from build123d import *

# Parameters (mm, degrees)
SKETCH1_W           = 2.54
SKETCH1_H           = 8.5
BOSS_EXTRUDE1_DEPTH = 1.52
SKETCH_1_W          = 0.8
SKETCH_1_H          = 1.54
CUT_EXTRUDE_1_DEPTH = 10.116166958
SKETCH2_W           = 0.8
SKETCH2_H           = 0.8
CUT_EXTRUDE1_DEPTH  = 7
CHAMFER_1_SIZE      = 0.4
BOSS_EXTRUDE2_DEPTH = 0.2
LPATTERN1_COUNT     = 3
LPATTERN1_PITCH     = 2.54


with BuildPart() as part:
    # Sketch1 → Boss-Extrude1 (new, symmetric)
    with BuildSketch(Plane(origin=(0, 0, 0), x_dir=(0, -1, 0), z_dir=(1, 0, 0))):
        with Locations((0, -4.25)):
            Rectangle(SKETCH1_W, SKETCH1_H)
    extrude(amount=BOSS_EXTRUDE1_DEPTH, both=True)

    # Эскиз1 → Вырез-Вытянуть1 (cut, through all)
    with BuildSketch(Plane(origin=(1.52, 0, 0), x_dir=(0, 0, -1), z_dir=(1, 0, 0))):
        with Locations((-0.4, 0)):
            Rectangle(SKETCH_1_W, SKETCH_1_H)
    extrude(amount=-CUT_EXTRUDE_1_DEPTH, mode=Mode.SUBTRACT)

    # Sketch2 → Cut-Extrude1 (cut)
    with BuildSketch(Plane(origin=(0, 0, 8.5), x_dir=(-1, 0, 0), z_dir=(0, 0, 1))):
        Rectangle(SKETCH2_W, SKETCH2_H)
    extrude(amount=-CUT_EXTRUDE1_DEPTH, mode=Mode.SUBTRACT)

    # Фаска1
    chamfer_1_edges = [part.edges().sort_by_distance(p)[0] for p in [
        (-0.4, 0, 8.5),
        (0, -0.4, 8.5),
        (0.4, 0, 8.5),
        (0, 0.4, 8.5),
    ]]
    chamfer(chamfer_1_edges, length=CHAMFER_1_SIZE)

    # Sketch3 → Boss-Extrude2 (add, symmetric)
    with BuildSketch(Plane(origin=(0, 0, 0), x_dir=(1, 0, 0), z_dir=(0, 1, 0))):
        Polygon((-0.3, 0), (-0.3, 1.7), (-0.15, 2.2), (0.15, 2.2), (0.3, 1.7), (0.3, 0), (0.3, -0.8), (-0.3, -0.8), align=None)
        Polygon((0.4, -1.5), (-0.4, -1.5), (-0.4, -6.9), (-0.3, -6.9), (-0.3, -1.6), (0.3, -1.6), (0.3, -6.9), (0.4, -6.9), align=None)
    extrude(amount=BOSS_EXTRUDE2_DEPTH, both=True)


with BuildPart() as lpattern1_1:
    # LPattern1: pattern copy
    add(part.part.moved(Location(Vector(1, 0, 0) * (1 * LPATTERN1_PITCH))))


with BuildPart() as lpattern1_2:
    # LPattern1: pattern copy
    add(part.part.moved(Location(Vector(1, 0, 0) * (2 * LPATTERN1_PITCH))))

    # Combine 1: union LPattern1_1, part
    add(lpattern1_1.part)
    add(part.part)


solid = lpattern1_2.part
Input: part model. Units: mm. Frame: model coordinates. A direction names the side the tool comes from. Give positions to 0.01 mm unless a question says otherwise; leave off trailing zeros. Loops run counter-clockwise (first coordinate to the right, second up) from the corner with the lowest first, then second, coordinate; pieces in that order, holes last. Notation, with made-up numbers: M 56.5,73 L 70.5,73 A15 cw 70.5,87 Z; hole C 37.5,32.5 d3. An arc over 180 degrees is marked long. Use CSV: the item, a comma, the result in double quotes.
(1) Material intervals for L1, parallel to X at y = 0.05, z = -0.75; L2, parallel to X at y = 0, z = 5.5; L3, parallel to Y at x = 3.75, z = 0.25, sorted ascending. Write a range as [from, to].
Outcome:
L1,"x = [-0.3, 0.3], [2.24, 2.84], [4.78, 5.38]"
L2,"x = [-1.52, -0.3], [0.3, 2.24], [2.84, 4.78], [5.38, 6.6]"
L3,"y = [-1.27, -0.77], [0.77, 1.27]"
(2) Section C-C, the plane x = 0. Return loops of the section in (y, z), plus the area to 3 significant figures.
Outcome:
outline,"M -1.27,0 L -0.77,0 L -0.77,0.8 L -0.2,0.8 L -0.2,-2.2 L 0.2,-2.2 L 0.2,0.8 L 0.77,0.8 L 0.77,0 L 1.27,0 L 1.27,8.5 L 0.8,8.5 L 0.4,8.1 L 0.4,1.5 L 0.2,1.5 L 0.2,1.6 L -0.2,1.6 L -0.2,1.5 L -0.4,1.5 L -0.4,8.1 L -0.8,8.5 L -1.27,8.5 Z"
area,"15.8 mm²"
(3) Set-up query: faces 5 (the face through (3, -1, 8.5)), 6 (the face through (5, -0.4, 5)). Return all of +Z, -Z, +X, -X, +Y, -Y with unobstructed straight access to the full face (end or side cutting, diameter ignored); none if empty.
Outcome:
face 5,"+Z, +X, -X, +Y, -Y"
face 6,"+Z"
(4) Section B-B, the plane y = 0.55. Return loops of the section in (x, z).
Outcome:
outline,"M -1.52,0.8 L 6.6,0.8 L 6.6,8.5 L 5.88,8.5 L 5.63,8.25 L 4.53,8.25 L 4.28,8.5 L 3.34,8.5 L 3.09,8.25 L 1.99,8.25 L 1.74,8.5 L 0.8,8.5 L 0.55,8.25 L -0.55,8.25 L -0.8,8.5 L -1.52,8.5 Z"
(5) Section A-A, the plane z = 7.75. Return loops of the section in (x, y).
Outcome:
outline,"M -1.52,-1.27 L 6.6,-1.27 L 6.6,1.27 L -1.52,1.27 Z; hole M -0.4,-0.4 L 0.4,-0.4 L 0.4,0.4 L -0.4,0.4 Z; hole M 2.14,-0.4 L 2.94,-0.4 L 2.94,0.4 L 2.14,0.4 Z; hole M 4.68,-0.4 L 5.48,-0.4 L 5.48,0.4 L 4.68,0.4 Z"
(6) Section D-D, the plane x = 4. Return loops of the section in (y, z), plus the area to 3 significant figures.
Outcome:
outline,"M -1.27,0 L -0.77,0 L -0.77,0.8 L 0.77,0.8 L 0.77,0 L 1.27,0 L 1.27,8.5 L -1.27,8.5 Z"
area,"20.4 mm²"
(7) Pull-direction query (X, two-part tool) for faces 1 (the face through (2.5, -0.4, 4.8)), 2 (the face through (-1.52, 0, 4)), 3 (the face through (3, -1.27, 4)), 4 (the face through (2.5, 0.4, 4.8)); classes: pulls with the +X half, pulls with the -X half, needs draft (parallel to the pull), parting line crosses it, or undercut.
Outcome:
face 1,"undercut"
face 2,"pulls with the -X half"
face 3,"needs draft"
face 4,"undercut"
